Autodesk Inventor part; units mm, degrees
ref_plane "Work Plane1" through (0, 0, -2.45) normal (0, 0, 1) x (1, 0, 0)
ref_plane "YZ Plane" through (0, 0, 0) normal (1, 0, 0) x (0, 1, 0)
ref_plane "XZ Plane" through (0, 0, 0) normal (0, 1, 0) x (-1, 0, 0)
sketch "Sketch1" plane through (0, 0, 0) normal (0, 1, 0) x (-1, 0, 0)
  circle A0 centre (0, 0) radius 2.45
  circle A1 centre (0, 0) radius 1.5
  dimension "d0" = 4.9
  dimension "d1" = 3
extrude "Extrusion1" add sketch "Sketch1" along normal mid plane 22.5
ref_plane "Work Plane1" through (0, 0, -2.45) normal (0, 0, 1) x (1, 0, 0)
sketch "Sketch2" plane through (0, 0, -2.45) normal (0, 0, 1) x (1, 0, 0)
  line L0 (2.5, 7.25) -> (-2.5, 7.25)
  line L1 (-2.5, 7.25) -> (-2.5, 1.25)
  line L2 (-2.5, 1.25) -> (2.5, 1.25)
  line L3 (2.5, 1.25) -> (2.5, 7.25)
  line L4 (2.45, 11.25) -> (-2.45, 11.25)
  point P0 (0, 0)
  point P1 (0, 7.25)
  dimension "d4" = 6
  dimension "d6" = 4
  dimension "d7" = 5
extrude "Extrusion2" cut sketch "Sketch2" along normal blind 0.5
properties part number "PulleyShaft"
Here's how the part is built. I have some questions about the finished solid (model axes, mm). Round coordinates to 2 decimals unless told otherwise and drop trailing zeros. Order: outer loops, then holes, each group sorted by start corner. A loop starts at its lowest first (then second) coordinate and runs counter-clockwise, first axis right, second up. Notation, with made-up numbers: M 70,-38.5 L 123,-38.5 A15 ccw 123,-9.5 Z; hole C 23,66 d10. An arc over 180 degrees is marked long. Answer in a Markdown table with one row per item.
Item 1: Imagine slicing it at A-A, the plane x = 0. Write out the boundary of the cut face in (y, z).
A:
| item | result |
|---|---|
| outline | M -11.25,-2.45 L 1.25,-2.45 L 1.25,-1.95 L 7.25,-1.95 L 7.25,-2.45 L 11.25,-2.45 L 11.25,-1.5 L -11.25,-1.5 Z; M -11.25,1.5 L 11.25,1.5 L 11.25,2.45 L -11.25,2.45 Z |
Item 2: I'm going to push flat-ended pins straight in: pin 1 (2 mm diameter, centred on x = -1, z = 1, fed in from -Y); pin 2 (2.5 mm diameter, centred on x = 0, z = 0, fed in from -Y); pin 3 (1.5 mm diameter, centred on y = -3.5, z = -1, fed in from -X); pin 4 (1.5 mm diameter, centred on x = 0.5, y = 5.5, fed in from -Z). Where does each tip first touch, or does it pass through?
A:
| item | result |
|---|---|
| pin 1 | stops at y = -11.25 |
| pin 2 | passes through |
| pin 3 | stops at x = -2.44 |
| pin 4 | stops at z = -1.95 |
Item 3: Imagine slicing it at C-C, the plane y = -7.5. Write out the boundary of the cut face in (x, z), and give its area (3 significant figures).
A:
| item | result |
|---|---|
| outline | C 0,0 d4.9; hole C 0,0 d3 |
| area | 11.8 mm2 |
Item 4: Thinking about a two-plate mould opening in Y: for faces 1 (the face through (0, 4, -1.95)), 2 (the face through (1.5, 0.16, 0.07)), 3 (the face through (0, 11.25, -2)), which applies, +Y half, -Y half, draft (parallel to the pull), parting line (faces both ways), or undercut?
A:
| item | result |
|---|---|
| face 1 | undercut |
| face 2 | draft |
| face 3 | +Y half |
Item 5: Imagine slicing it at B-B, the plane z = 0. Write out the boundary of the cut face in (x, y), and give its area (4 significant figures).
A:
| item | result |
|---|---|
| outline | M -2.45,-11.25 L -1.5,-11.25 L -1.5,11.25 L -2.45,11.25 Z; M 1.5,-11.25 L 2.45,-11.25 L 2.45,11.25 L 1.5,11.25 Z |
| area | 42.75 mm2 |
Item 6: Imagine slicing it at D-D, the plane x = 1.05. Write out the boundary of the cut face in (y, z).
A:
| item | result |
|---|---|
| outline | M -11.25,-2.21 L 1.25,-2.21 L 1.25,-1.95 L 7.25,-1.95 L 7.25,-2.21 L 11.25,-2.21 L 11.25,-1.07 L -11.25,-1.07 Z; M -11.25,1.07 L 11.25,1.07 L 11.25,2.21 L -11.25,2.21 Z |
Item 7: If I drill on L1, parallel to Y at x = -0.95, z = -2.1; L2, parallel to Z at x = 0, y = -3; L3, parallel to Z at x = 0, y = 4.5, over which ranges is the centre line in solid material (lowest first)? Write a range as from..to.
A:
| item | result |
|---|---|
| L1 | y = -11.25..1.25, 7.25..11.25 |
| L2 | z = -2.45..-1.5, 1.5..2.45 |
| L3 | z = -1.95..-1.5, 1.5..2.45 |
